```python
from build123d import *

# Parameters (mm, degrees)
F0_R      = 7.62
F1_DEPTH  = 27.94
F2_R      = 4.292472
F3_R      = 4.292472
F1_FACE_R = 3.327528
F4_DEPTH  = 12.7
F5_R      = 3.81
F6_DEPTH  = 2.54
F7_SIZE   = 1.016
F8_R      = 1.905
F9_DEPTH  = 43.18


with BuildPart() as f1:
    # F0 (on Top) → F1 (new body)
    with BuildSketch(Plane.XY):
        Circle(F0_R)
    extrude(amount=F1_DEPTH)

    # F2
    f2_edges = [f1.edges().sort_by_distance(p)[0] for p in [
        (-7.62, 0, 0),
    ]]
    fillet(f2_edges, radius=F2_R)

    # F3
    f3_edges = [f1.edges().sort_by_distance(p)[0] for p in [
        (-7.62, 0, 27.94),
    ]]
    fillet(f3_edges, radius=F3_R)

    # F1_face (on face) → F4 (join)
    with BuildSketch(Plane.XY.offset(27.94)):
        Circle(F1_FACE_R)
    extrude(amount=F4_DEPTH)

    # F5 (on face) → F6 (join)
    with BuildSketch(Plane.XY.offset(40.64)):
        Circle(F5_R)
    extrude(amount=F6_DEPTH)

    # F7
    f7_edges = [f1.edges().sort_by_distance(p)[0] for p in [
        (-3.81, 0, 43.18),
    ]]
    chamfer(f7_edges, length=F7_SIZE)

    # F8 (on face) → F9 (cut)
    with BuildSketch(Plane.XY.offset(43.18)):
        Circle(F8_R)
    extrude(amount=-F9_DEPTH, mode=Mode.SUBTRACT)


solid = f1.part
```
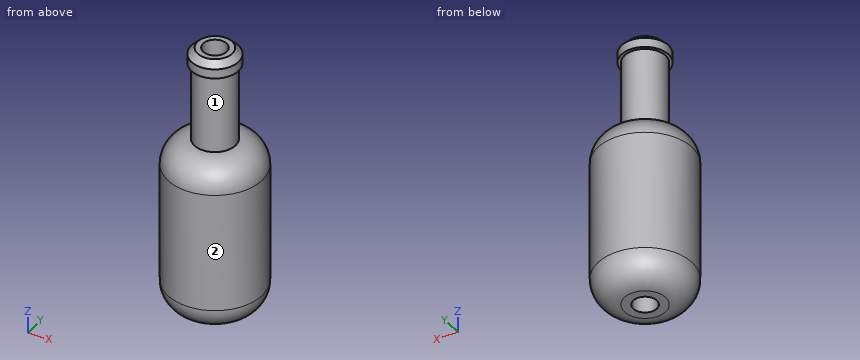
Geometry check sheet. Reference: the model listing, model coordinates, mm. Face numbers are marked on the shaded views. Give positions to 0.01 mm unless a question says otherwise; leave off trailing zeros. Write item = value, one per line. Start each with the question number.
1) Draft check along Z on the marked faces 1 and 2. Enter one of: released by +Z, released by -Z, zero draft, split by the parting line, or undercut.
2) Scan lines: L1, parallel to Y at x = 0, z = 16.5 (3 decimals); L2, parallel to X at y = -0.25, z = 28; L3, parallel to Y at x = 0, z = 31 (3 decimals). Record each from-to range of solid material in increasing order.
3) Gauge pin test, flat ends, axial feed: pin 1 Ø1.5 at (y, z) = (-5, 23) entering from +X; pin 2 Ø6 at (y, z) = (-4, 9.5) entering from +X; pin 3 Ø5 at (y, z) = (-6, 5.5) entering from +X; pin 4 Ø2.5 at (x, y) = (0, 0) entering from -Z. Record the tip position at first contact, or that the pin passes through.
Geometry check:
q1.face_1 = undercut
q1.face_2 = zero draft
q2.L1 = -7.62 to -1.905, 1.905 to 7.62
q2.L2 = -3.32 to -1.89, 1.89 to 3.32
q2.L3 = -3.328 to -1.905, 1.905 to 3.328
q3.pin_1 = 6.32
q3.pin_2 = 7.55
q3.pin_3 = 6.77
q3.pin_4 = through
